For this review, use the dimensioned drawing (mm, ordinates from the lowest corner) and the shaded views. Coordinates: 2 decimals unless noted, no trailing zeros. Loops run counter-clockwise (first coordinate to the right, second up) from the corner with the lowest first, then second, coordinate; pieces in that order, holes last. Notation, with made-up numbers: (36, -27) -> (43, -27) arc R11 ccw to (43, -13) -> close; hole circle Ø9 at (9.25, 40). An arc over 180 degrees is marked (long way). Answer as a JSON object with one key per item and string values.
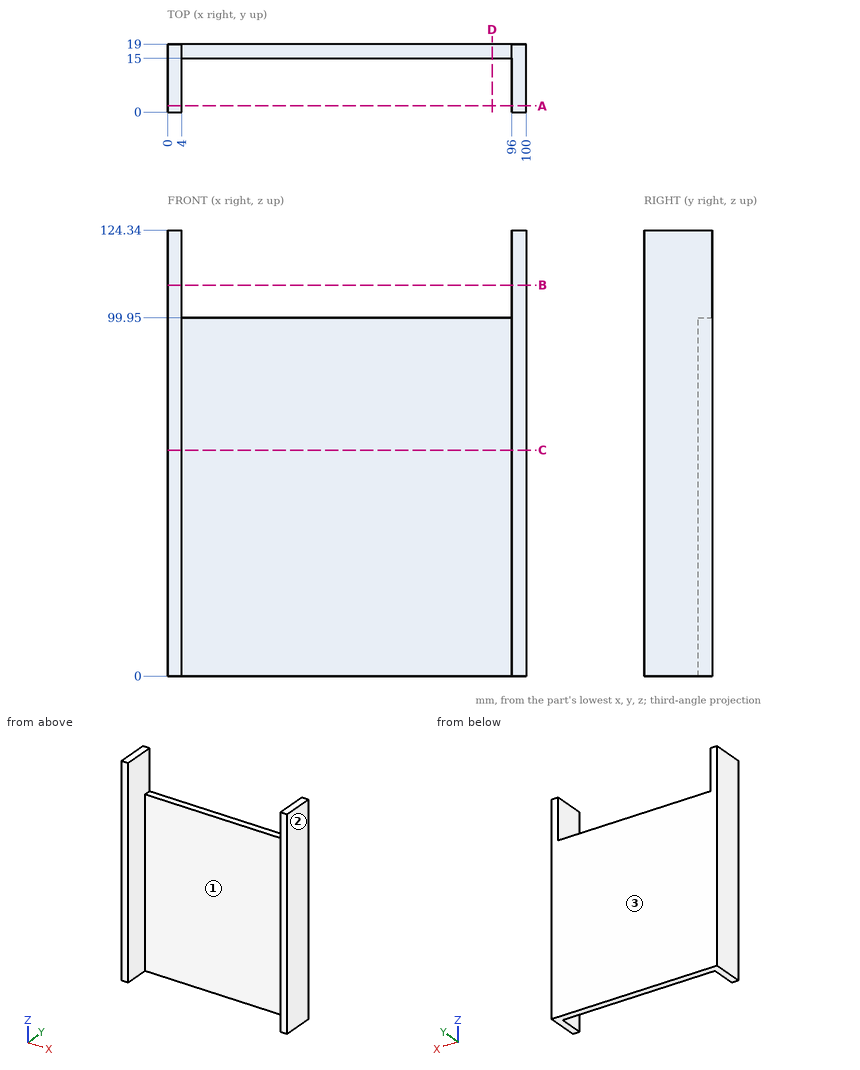
1) Add section D-D, the plane x = 90.5. Give the boundary of the cut face in (y, z).
Completed:
{"outline": "(15, 0) -> (19, 0) -> (19, 99.95) -> (15, 99.95) -> close"}
2) The part is to be moulded in two halves that separate along X. For the marked faces 1, 2 and 3, say which applies: pulls with the +X half, pulls with the -X half, needs draft (parallel to the pull), parting line crosses it, or undercut.
Completed:
{"face 1": "undercut", "face 2": "pulls with the +X half", "face 3": "needs draft"}
3) Add section B-B, the plane z = 109. Give the boundary of the cut face in (x, y), and give its area (3 significant figures).
Completed:
{"outline": "(0, 0) -> (4, 0) -> (4, 19) -> (0, 19) -> close; (96, 0) -> (100, 0) -> (100, 19) -> (96, 19) -> close", "area": "152 mm²"}
4) Clearance check with flat-ended pins moving along their axes: pin 1 Ø3 at (x, y) = (52, 17) entering from +Z; pin 2 Ø1 at (x, z) = (44, 94.5) entering from -Y. State where each tip first meets the part, or that it passes through.
Completed:
{"pin 1": "z = 99.95", "pin 2": "y = 15"}
5) Wall thickness on probe 1 along X at (y, z) = (6.75, 90); probe 2 along Y at (x, z) = (89.5, 61.5); probe 3 along Z at (x, y) = (44.5, 16.5): over which ranges is each line inside the solid? List them lowest first.
Completed:
{"probe 1": "0 to 4, 96 to 100", "probe 2": "15 to 19", "probe 3": "0 to 99.95"}
6) Add section C-C, the plane z = 63. Give the boundary of the cut face in (x, y).
Completed:
{"outline": "(0, 0) -> (4, 0) -> (4, 15) -> (96, 15) -> (96, 0) -> (100, 0) -> (100, 19) -> (0, 19) -> close"}
7) Add section A-A, the plane y = 1.75. Give the boundary of the cut face in (x, z), and give its area (3 significant figures).
Completed:
{"outline": "(0, 0) -> (4, 0) -> (4, 124.34) -> (0, 124.34) -> close; (96, 0) -> (100, 0) -> (100, 124.34) -> (96, 124.34) -> close", "area": "995 mm²"}
